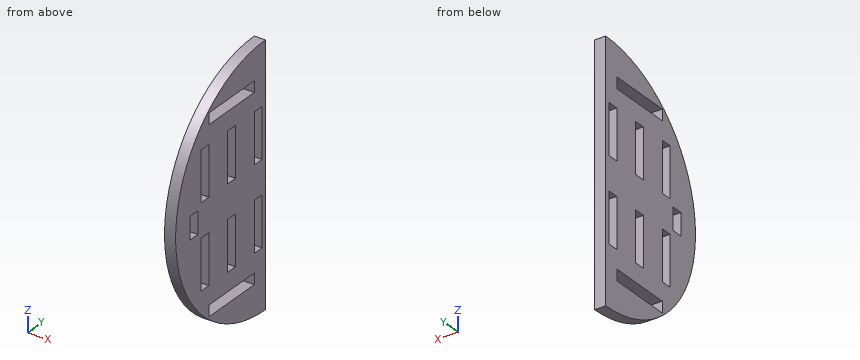
```python
from build123d import *

# Parameters (mm, degrees)
SKETCH1_W           = 22.5
SKETCH1_H           = 5
SKETCH1_W_2         = 10
SKETCH1_W_3         = 5
SKETCH1_H_2         = 29
BOSS_EXTRUDE1_DEPTH = 5


with BuildPart() as part:
    # Sketch1 → Boss-Extrude1 (new body)
    with BuildSketch(Plane(origin=(0, 0, 0), x_dir=(0, 0, -1), z_dir=(1, 0, 0))):
        with BuildLine():
            Line((57.224821465, 0), (-57.224821465, 0))
            ThreePointArc((-57.224821465, 0), (0, -57.224821465), (57.224821465, 0))
        make_face()
        with Locations((-18.75, -38.548791642)):
            Rectangle(SKETCH1_W, SKETCH1_H, mode=Mode.SUBTRACT)
        with Locations((0, -45.5)):
            Rectangle(SKETCH1_W_2, SKETCH1_H, mode=Mode.SUBTRACT)
        with Locations((18.75, -38.548791642)):
            Rectangle(SKETCH1_W, SKETCH1_H, mode=Mode.SUBTRACT)
        with Locations((-40.75, -21.548791642)):
            Rectangle(SKETCH1_W_3, SKETCH1_H_2, mode=Mode.SUBTRACT)
        with Locations((-18.75, -21.548791642)):
            Rectangle(SKETCH1_W, SKETCH1_H, mode=Mode.SUBTRACT)
        with Locations((-18.75, -4.548791642)):
            Rectangle(SKETCH1_W, SKETCH1_H, mode=Mode.SUBTRACT)
        with Locations((40.75, -21.548791642)):
            Rectangle(SKETCH1_W_3, SKETCH1_H_2, mode=Mode.SUBTRACT)
        with Locations((18.75, -21.548791642)):
            Rectangle(SKETCH1_W, SKETCH1_H, mode=Mode.SUBTRACT)
        with Locations((18.75, -4.548791642)):
            Rectangle(SKETCH1_W, SKETCH1_H, mode=Mode.SUBTRACT)
    extrude(amount=BOSS_EXTRUDE1_DEPTH)


solid = part.part
```
Build history of the part. All positions in model axes, mm. Round coordinates to 2 decimals unless told otherwise and drop trailing zeros. Write each loop counter-clockwise with the first axis right and the second up, starting at its lowest first coordinate (ties: lowest second). Pieces come first, ordered by that corner, then holes.
1) Band-saw the part on C-C, the plane y = -27. List the corners of the cut face in (x, z).
2) Pin check, flat tips, straight feed: pin 1 (2.5 mm diameter, centred on x = 2, z = -24, fed in from -Y); pin 2 (1.5 mm diameter, centred on x = 3, y = -38.5, fed in from -Z); pin 3 (1.5 mm diameter, centred on x = 1.5, y = -21, fed in from -Z); pin 4 (5 mm diameter, centred on y = -28, z = -38.5, fed in from +X). Stop position of each tip, or through.
3) Band-saw the part on B-B, the plane y = -21. List the corners of the cut face in (x, z), and give its area (3 significant figures).
4) Band-saw the part on A-A, the plane z = 0. List the corners of the cut face in (x, y), and give its area (3 significant figures).
5) Band-saw the part on D-D, the plane z = -19. List the corners of the cut face in (x, y), and give its area (3 significant figures).
6) Drill centre lines: probe 1 along Z at (x, y) = (1, -28); probe 2 along Z at (x, y) = (0.3, -8); probe 3 along Y at (x, z) = (2.2, -11). Where is each one in solid material? Low to high.
Ans:
1. outline: (0, -50.45) - (5, -50.45) - (5, -43.25) - (0, -43.25) - close; (0, -38.25) - (5, -38.25) - (5, 38.25) - (0, 38.25) - close; (0, 43.25) - (5, 43.25) - (5, 50.45) - (0, 50.45) - close
2. pin 1: stops at y = -52.51
2. pin 2: stops at z = -43.01
2. pin 3: stops at z = -53.52
2. pin 4: stops at x = 5
3. outline: (0, -53.23) - (5, -53.23) - (5, -43.25) - (0, -43.25) - close; (0, -38.25) - (5, -38.25) - (5, -30) - (0, -30) - close; (0, -7.5) - (5, -7.5) - (5, 7.5) - (0, 7.5) - close; (0, 30) - (5, 30) - (5, 38.25) - (0, 38.25) - close; (0, 43.25) - (5, 43.25) - (5, 53.23) - (0, 53.23) - close
3. area: 257 mm2
4. outline: (0, -57.22) - (5, -57.22) - (5, -48) - (0, -48) - close; (0, -43) - (5, -43) - (5, 0) - (0, 0) - close
4. area: 261 mm2
5. outline: (0, -53.98) - (5, -53.98) - (5, -41.05) - (0, -41.05) - close; (0, -36.05) - (5, -36.05) - (5, -24.05) - (0, -24.05) - close; (0, -19.05) - (5, -19.05) - (5, -7.05) - (0, -7.05) - close; (0, -2.05) - (5, -2.05) - (5, 0) - (0, 0) - close
5. area: 195 mm2
6. probe 1: z = -49.91 to -43.25, -38.25 to 38.25, 43.25 to 49.91
6. probe 2: z = -56.66 to -43.25, -38.25 to 38.25, 43.25 to 56.66
6. probe 3: y = -56.16 to -41.05, -36.05 to -24.05, -19.05 to -7.05, -2.05 to 0
